Work out the finished part from the listing and answer in its coordinate system (mm). A direction names the side the tool comes from. Round coordinates to 2 decimals unless told otherwise and drop trailing zeros. Write each loop counter-clockwise with the first axis right and the second up, starting at its lowest first coordinate (ties: lowest second). Pieces come first, ordered by that corner, then holes.
from build123d import *

# Parameters (mm, degrees)
SKETCH1_W                = 35.8
SKETCH1_H                = 12
BOARD_DEPTH              = 1.6
SKETCH2_R                = 1.575
HOLE_DEPTH               = 2.6
SKETCH3_W                = 5.9
SKETCH3_H                = 3.82
SETUP_SWITCH_DEPTH       = 2.7
SURFACE_START            = -3.4
SKETCH4_W                = 0.5
SKETCH4_H                = 0.5
SURFACE_CONNECTORS_DEPTH = 5.9
LPATTERN1_COUNT          = 6
LPATTERN1_PITCH          = 2
LPATTERN1_COUNT_DIR2     = 2
LPATTERN1_PITCH_DIR2     = 2
SKETCH5_W                = 4
SKETCH5_H                = 3.8
CONNECTOR_BODY_DEPTH     = 12
SKETCH6_W                = 0.5
SKETCH6_H                = 0.5
CONNECTOR_PIN_DEPTH      = 3.8
LPATTERN2_COUNT          = 6
LPATTERN2_PITCH          = 2
LPATTERN2_COUNT_DIR2     = 2
LPATTERN2_PITCH_DIR2     = 2


with BuildPart() as part:
    # Sketch1 → Board (new body)
    with BuildSketch(Plane(origin=(0, 0, 0), x_dir=(1, 0, 0), z_dir=(0, 1, 0))):
        Rectangle(SKETCH1_W, SKETCH1_H)
    extrude(amount=BOARD_DEPTH)

    # Sketch2 → Hole (cut, through all)
    with BuildSketch(Plane(origin=(0, 1.6, 0), x_dir=(-1, 0, 0), z_dir=(0, 1, 0))):
        with Locations(Location((-15.625, 3.575, 0), (0, 0, 90))):  # turned: the seam where the file's is
            Circle(SKETCH2_R)
    extrude(amount=-HOLE_DEPTH, mode=Mode.SUBTRACT)

    # Sketch3 → Setup Switch (add)
    with BuildSketch(Plane(origin=(0, 1.6, 0), x_dir=(-1, 0, 0), z_dir=(0, 1, 0))):
        with Locations((-13.15, -3.64)):
            Rectangle(SKETCH3_W, SKETCH3_H)
    extrude(amount=SETUP_SWITCH_DEPTH)

    # Sketch4 → Surface Connectors (add)
    with BuildSketch(Plane(origin=(0, 1.6, 0), x_dir=(-1, 0, 0), z_dir=(0, 1, 0)).offset(SURFACE_START)):
        with Locations((17.15, 5.25)):
            Rectangle(SKETCH4_W, SKETCH4_H)
    surface_connectors = extrude(amount=SURFACE_CONNECTORS_DEPTH)

    # LPattern1: Surface Connectors 6 × 2
    with Locations(*[(j * LPATTERN1_PITCH_DIR2, 0, -i * LPATTERN1_PITCH) for i in range(LPATTERN1_COUNT) for j in range(LPATTERN1_COUNT_DIR2) if (i, j) != (0, 0)]):
        add(surface_connectors)

    # Sketch5 → Connector Body (add)
    with BuildSketch(Plane.XY.offset(6)):
        with Locations((-17, 4)):
            Rectangle(SKETCH5_W, SKETCH5_H)
    extrude(amount=-CONNECTOR_BODY_DEPTH)

    # Sketch6 → Connector Pin (add)
    with BuildSketch(Plane.ZY.offset(19)):
        with Locations((5.25, 5.15)):
            Rectangle(SKETCH6_W, SKETCH6_H)
    connector_pin = extrude(amount=CONNECTOR_PIN_DEPTH)

    # LPattern2: Connector Pin 6 × 2
    with Locations(*[(0, -j * LPATTERN2_PITCH_DIR2, -i * LPATTERN2_PITCH) for i in range(LPATTERN2_COUNT) for j in range(LPATTERN2_COUNT_DIR2) if (i, j) != (0, 0)]):
        add(connector_pin)


solid = part.part
Q1. Find section A-A (z = -4). Determine the outline of the cut face in (x, y), plus the area to 3 significant figures.
Q2. A tool of negligible diameter and unlimited length cuts with its end or side. For faces 1 (the face through (-17.9, 1, 0)), 2 (the face through (13, 4.3, -4)), 3 (the face through (-17, 2.1, 0)), 4 (the face through (13, 3, -1.73)), 5 (the face through (10.2, 3, -4)), from which of +Z, -Z, +X, -X, +Y, -Y can it reach the whole face along a straight path? Write none if from no direction.
Q3. Find the intervals of material crossed by L1, parallel to X at y = 4.25, z = -5.5; L2, parallel to Z at x = 15.5, y = 1.75; L3, parallel to X at y = 4.5, z = 1.5, in increasing order.
Q4. Find section C-C (z = 0.5). Determine the outline of the cut face in (x, y).
Q5. Find section D-D (y = -1). Count the separate pieces of the cut face and the enclosed holes in it, plus the area to 3 significant figures.
Q6. Given pin 1 (2 mm diameter, centred on y = 3.5, z = 2.5, fed in from +X); pin 2 (5 mm diameter, centred on x = -1.5, z = -4, fed in from -Y); pin 3 (5 mm diameter, centred on x = 9, z = -4, fed in from +Y), each flat-ended and moving along its own axis, determine where each tip first touches the part or whether it passes through.
Q7. The mould has two halves that part along Z. Classify faces 6 (the face through (13, 3, -5.55)), 7 (the face through (-15, 4, 0)), 8 (the face through (-17, 4, 6)), 9 (the face through (17.9, 1, 0)): +Z half, -Z half, draft (parallel to the pull), parting line (faces both ways), or undercut.
Report:
1. outline: (-19, 2.1) - (-15, 2.1) - (-15, 5.9) - (-19, 5.9) - close; (-17.9, 0) - (17.9, 0) - (17.9, 1.6) - (16.1, 1.6) - (16.1, 4.3) - (10.2, 4.3) - (10.2, 1.6) - (-17.9, 1.6) - close
1. area: 88.4 mm2
2. face 1: +Z, -Z, -X, -Y
2. face 2: +Z, -Z, +X, +Y
2. face 3: none
2. face 4: +Z, +X, +Y
2. face 5: +Z, -Z, +Y
3. L1: x = -19 to -15, 10.2 to 16.1
3. L2: z = -5.55 to -1.73
3. L3: x = -19 to -15
4. outline: (-19, 2.1) - (-15, 2.1) - (-15, 5.9) - (-19, 5.9) - close; (-17.9, 0) - (17.9, 0) - (17.9, 1.6) - (-17.9, 1.6) - close
5. separate pieces: 12
5. enclosed holes: 0
5. area: 3.00 mm2
6. pin 1: stops at x = -14.9
6. pin 2: stops at y = 0
6. pin 3: stops at y = 4.3
7. face 6: -Z half
7. face 7: undercut
7. face 8: +Z half
7. face 9: draft
